```python
from build123d import *

# Parameters (mm, degrees)
F0_W         = 20
F0_H         = 30
F0_R         = 6.15
F1_DEPTH     = 4
F1_FACE_W    = 20
F1_FACE_H    = 30
F1_FACE_R    = 6.15
F0_R_2       = 2
F2_DEPTH     = 0.5
F3_W         = 20
F3_H         = 10
F4_DEPTH     = 5
F5_R         = 3.25
F6_DEPTH     = 25
F7_T1_DEPTH  = 97.9025398997
F8_R         = 9.99999
F9_R         = 1
F10_DEPTH    = 25
F11_T1_DEPTH = 45


# Not quite as in the source:
# - a fillet or chamfer that OpenCascade refuses, or shapes differently, is made with other operations: its cross-section is extruded or revolved along the edge and cut away or added
# - a fillet or chamfer is up to 0.001 mm smaller than in the source, because OpenCascade refuses the exact size
# - a feature names something its author has since deleted; it is built from what else it names


with BuildPart() as f1:
    # F0 (on Top) → F1 (new body)
    with BuildSketch(Plane.XY):
        with Locations((10, 15)):
            Rectangle(F0_W, F0_H)
        with Locations((10, 20)):
            Circle(F0_R, mode=Mode.SUBTRACT)
    extrude(amount=F1_DEPTH)

    # F1_face (on face) + F0 (on Top) → F2 (join)
    with BuildSketch(Plane(origin=(10, 13.7652894827, 4), x_dir=(1, 0, 0), z_dir=(0, 0, 1))):
        with Locations((0, 1.2347105173)):
            Rectangle(F1_FACE_W, F1_FACE_H)
        with Locations((0, 6.2347105173)):
            Circle(F1_FACE_R, mode=Mode.SUBTRACT)
    with BuildSketch(Plane.XY):
        with Locations((10, 20)):
            Circle(F0_R)
        with Locations((10, 20)):
            Circle(F0_R_2, mode=Mode.SUBTRACT)
    extrude(amount=F2_DEPTH)

    # F3 (on face) → F4 (join)
    with BuildSketch(Plane.XY.offset(4.5)):
        with Locations((10, 5)):
            Rectangle(F3_W, F3_H)
    extrude(amount=F4_DEPTH)

    # F5 (on face) → F6 (cut)
    with BuildSketch(Plane(origin=(0, 0, 0), x_dir=(0, -1, 0), z_dir=(-1, 0, 0))):
        with Locations((-5, 5)):
            Circle(F5_R)
    extrude(amount=-F6_DEPTH, mode=Mode.SUBTRACT)

    # F7: chamfer of 4 x 15 on 1 edges, made by hand

    # F7_s2 → F7_t1 (cut)
    with BuildSketch(Plane.YZ.offset(-38.9512699498)):
        Polygon((30, 0.5), (15, 4.5), (30, 4.5), align=None)
    extrude(amount=F7_T1_DEPTH, mode=Mode.SUBTRACT)

    # F8 (radius 10 in the source; OpenCascade refuses exactly that, so slightly less here)
    f8_edges = [f1.edges().sort_by_distance(p)[0] for p in [
        (0, 30, 0.25),
        (20, 30, 0.25),
    ]]
    fillet(f8_edges, radius=F8_R)

    # F9 (on face) → F10 (cut)
    with BuildSketch(Plane.XY.offset(9.5)):
        with Locations((4, 5)):
            Circle(F9_R)
        with Locations((16, 5)):
            Circle(F9_R)
    extrude(amount=-F10_DEPTH, mode=Mode.SUBTRACT)

    # F11: fillet of radius 5 on 2 edges, made by hand

    # F11_s2 → F11_t1 (cut)
    with BuildSketch(Plane.YZ.offset(-12.5)):
        with BuildLine():
            ThreePointArc((0, 4.5), (1.4644660941, 8.0355339059), (5, 9.5))
            Line((5, 9.5), (0, 9.5))
            Line((0, 9.5), (0, 4.5))
        make_face()
        with BuildLine():
            ThreePointArc((5, 9.5), (8.5355339059, 8.0355339059), (10, 4.5))
            Line((10, 4.5), (10, 9.5))
            Line((10, 9.5), (5, 9.5))
        make_face()
    extrude(amount=F11_T1_DEPTH, mode=Mode.SUBTRACT)


solid = f1.part
```
Work out the finished part from the listing and answer in its coordinate system (mm). A direction names the side the tool comes from. Give positions to 0.01 mm unless a question says otherwise; leave off trailing zeros. Order: outer loops, then holes, each group sorted by start corner. A loop starts at its lowest first (then second) coordinate and runs counter-clockwise, first axis right, second up.
1. Section A-A, the plane y = 3 is taken. Determine the outline of the cut face in (x, z).
Result sheet:
outline: (0, 0) - (20, 0) - (20, 2.44) - (0, 2.44) - close; (0, 7.56) - (20, 7.56) - (20, 9.08) - (0, 9.08) - close
2. Each of these flat-tipped pins is pushed along its axis until it touches: P1, Ø1, axis at x = 2, z = 7.5, coming from the +Y side; P2, Ø3, axis at x = 11.5, y = 26, coming from the +Z side; P3, Ø2.5, axis at x = 4, y = 5, coming from the +Z side; P4, Ø6, axis at x = 8, y = 23, coming from the +Z side. Where does it stop, or does it pass through?
Result sheet:
P1: stops at y = 9.33
P2: stops at z = 1.72
P3: stops at z = 9.5
P4: stops at z = 2.18
3. For faces 4 (the flat face through (20, 10, 3)), 5 (the flat face through (10, 13, 4.5)), 6 (the flat face through (13, 20, 0.5)), determine the directions among +Z, -Z, +X, -X, +Y, -Y from which every point of the face is accessible in a straight line to the end or side of a thin tool.
Result sheet:
face 4: +Z, -Z, +X, +Y, -Y
face 5: +Z, +X, -X, +Y
face 6: +Z
4. The mould has two halves that part along Z. Classify faces 1 (the cylindrical face through (9.86, 3.5, 2.117)), 2 (the flat face through (7.638, 25.938, 1.583)), 3 (the cylindrical face through (15.263, 5.676, 8.806)): released by +Z, released by -Z, zero draft, split by the parting line, or undercut.
Result sheet:
face 1: undercut
face 2: released by +Z
face 3: zero draft
5. Section C-C, the plane x = 4.5 is taken. Determine the outline of the cut face in (y, z), and give its area (3 significant figures).
Result sheet:
outline: (0, 0) - (4.13, 0) - (4.13, 1.87) arc R3.25 cw to (4.13, 8.13) - (4.13, 9.42) arc R5 ccw to (0, 4.5) - close; (5.87, 0) - (28.35, 0) - (28.35, 0.94) - (22.75, 2.43) - (22.75, 0.5) - (17.25, 0.5) - (17.25, 3.9) - (15, 4.5) - (10, 4.5) arc R5 ccw to (5.87, 9.42) - (5.87, 8.13) arc R3.25 cw to (5.87, 1.87) - close
area: 89.9 mm2
6. Section D-D, the plane y = 24 is taken. Determine the outline of the cut face in (x, z).
Result sheet:
outline: (0.83, 0) - (19.17, 0) - (19.17, 2.1) - (14.67, 2.1) - (14.67, 0.5) - (5.33, 0.5) - (5.33, 2.1) - (0.83, 2.1) - close
7. Section B-B, the plane z = 5.5 is taken. Determine the outline of the cut face in (x, y).
Result sheet:
outline: (0, 0.1) - (20, 0.1) - (20, 1.79) - (0, 1.79) - close; (0, 8.21) - (20, 8.21) - (20, 9.9) - (0, 9.9) - close
8. Straight lines are drawn through the part: L1, parallel to X at y = 5, z = 1.2; L2, parallel to X at y = 20, z = 1.5; L3, parallel to Y at x = 12.5, z = 3.75. For each, find the intervals that lie inside material, in ascending order.
Result sheet:
L1: x = 0 to 3, 5 to 15, 17 to 20
L2: x = 0 to 3.85, 16.15 to 20
L3: y = 0 to 2, 8 to 14.38
